The model under review builds one solid part; all positions refer to its coordinate system, in mm. Face numbers are marked on the shaded views. A direction names the side the tool comes from. Give positions to 0.01 mm unless a question says otherwise; leave off trailing zeros. Write each loop counter-clockwise with the first axis right and the second up, starting at its lowest first coordinate (ties: lowest second). Pieces come first, ordered by that corner, then holes. Notation, with made-up numbers: (0.25, 9.25) - (39.25, 9.25) arc R27 ccw to (39.25, 31.25) - close; hole circle Ø7 at (75, 18). An arc over 180 degrees is marked (long way). Write item = value, one per line.
```python
from build123d import *

# Parameters (mm, degrees)
F0_W      = 50.8
F0_H      = 31.75
F1_DEPTH  = 57.15
F2_W      = 50.8
F2_H      = 25.4
F3_DEPTH  = 19.05
F5_DEPTH  = 19.05
F6_DEPTH  = 6.35
F8_DEPTH  = 57.151
F10_DEPTH = 12.701
F12_DEPTH = 12.701
F14_DEPTH = 25.4


with BuildPart() as f1:
    # F0 (on Top) → F1 (new body)
    with BuildSketch(Plane.XY):
        with Locations((25.4, 15.875)):
            Rectangle(F0_W, F0_H)
    extrude(amount=F1_DEPTH)

    # F2 (on face) → F3 (cut)
    with BuildSketch(Plane.XZ):
        with Locations((25.4, 19.05)):
            Rectangle(F2_W, F2_H)
    extrude(amount=-F3_DEPTH, mode=Mode.SUBTRACT)

    # F4 (on face) → F5 (cut)
    with BuildSketch(Plane.XZ):
        with BuildLine():
            ThreePointArc((12.7, 44.45), (16.4197438789, 53.4302561211), (25.4, 57.15))
            Line((25.4, 57.15), (0, 57.15))
            Line((0, 57.15), (0, 44.45))
            Line((0, 44.45), (12.7, 44.45))
        make_face()
        with BuildLine():
            Line((0, 31.75), (25.4, 31.75))
            ThreePointArc((25.4, 31.75), (16.4197438789, 35.4697438789), (12.7, 44.45))
            Line((12.7, 44.45), (0, 44.45))
            Line((0, 44.45), (0, 31.75))
        make_face()
        with BuildLine():
            Line((50.8, 44.45), (38.1, 44.45))
            ThreePointArc((38.1, 44.45), (34.3802561211, 35.4697438789), (25.4, 31.75))
            Line((25.4, 31.75), (50.8, 31.75))
            Line((50.8, 31.75), (50.8, 44.45))
        make_face()
        with BuildLine():
            ThreePointArc((25.4, 57.15), (34.3802561211, 53.4302561211), (38.1, 44.45))
            Line((38.1, 44.45), (50.8, 44.45))
            Line((50.8, 44.45), (50.8, 57.15))
            Line((50.8, 57.15), (25.4, 57.15))
        make_face()
        with BuildLine():
            Line((19.05, 44.45), (31.75, 44.45))
            ThreePointArc((31.75, 44.45), (25.4, 50.8), (19.05, 44.45))
        make_face()
        with BuildLine():
            ThreePointArc((19.05, 44.45), (25.4, 38.1), (31.75, 44.45))
            Line((31.75, 44.45), (19.05, 44.45))
        make_face()
    extrude(amount=-F5_DEPTH, mode=Mode.SUBTRACT)

    # F6 (cut): a face of the model
    f6_faces = [f1.faces().sort_by_distance(p)[0] for p in [
        (25.4, 0, 56.7907897552),
    ]]
    extrude(f6_faces, amount=-F6_DEPTH, mode=Mode.SUBTRACT)

    # F7 (on face) → F8 (cut, through all)
    with BuildSketch(Plane(origin=(0, 0, 0), x_dir=(1, 0, 0), z_dir=(0, 0, -1))):
        with BuildLine():
            Line((0, 0), (0, -12.7))
            ThreePointArc((0, -12.7), (3.7197438789, -3.7197438789), (12.7, 0))
            Line((12.7, 0), (0, 0))
        make_face()
        with BuildLine():
            Line((50.8, 0), (38.1, 0))
            ThreePointArc((38.1, 0), (47.0802561211, -3.7197438789), (50.8, -12.7))
            Line((50.8, -12.7), (50.8, 0))
        make_face()
    extrude(amount=-F8_DEPTH, mode=Mode.SUBTRACT)

    # F9 (on face) → F10 (cut, through all)
    with BuildSketch(Plane.XZ.offset(-19.05)):
        Polygon((12.7, 44.45), (12.7, 57.15), (0, 57.15), (0, 19.05), (12.7, 19.05), align=None)
        Polygon((50.8, 57.15), (38.1, 57.15), (38.1, 44.45), (38.1, 19.05), (50.8, 19.05), align=None)
        with BuildLine():
            Line((38.1, 57.15), (25.4, 57.15))
            ThreePointArc((25.4, 57.15), (34.3802561211, 53.4302561211), (38.1, 44.45))
            Line((38.1, 44.45), (38.1, 57.15))
        make_face()
        with BuildLine():
            Line((25.4, 57.15), (12.7, 57.15))
            Line((12.7, 57.15), (12.7, 44.45))
            ThreePointArc((12.7, 44.45), (16.4197438789, 53.4302561211), (25.4, 57.15))
        make_face()
    extrude(amount=-F10_DEPTH, mode=Mode.SUBTRACT)

    # F11 (on face) → F12 (cut, through all)
    with BuildSketch(Plane.XZ.offset(-19.05)):
        with BuildLine():
            Line((0, 19.05), (0, 6.35))
            ThreePointArc((0, 6.35), (8.9802561211, 10.0697438789), (12.7, 19.05))
            Line((12.7, 19.05), (0, 19.05))
        make_face()
        with BuildLine():
            ThreePointArc((38.1, 19.05), (41.8197438789, 10.0697438789), (50.8, 6.35))
            Line((50.8, 6.35), (50.8, 19.05))
            Line((50.8, 19.05), (38.1, 19.05))
        make_face()
    extrude(amount=-F12_DEPTH, mode=Mode.SUBTRACT)

    # F13 (on face) → F14 (cut)
    with BuildSketch(Plane(origin=(0, 0, 0), x_dir=(1, 0, 0), z_dir=(0, 0, -1))):
        with BuildLine():
            Line((9.525, -9.525), (6.35, -9.525))
            ThreePointArc((6.35, -9.525), (9.525, -12.7), (12.7, -9.525))
            ThreePointArc((12.7, -9.525), (11.7700640303, -7.2799359697), (9.525, -6.35))
            Line((9.525, -6.35), (9.525, -9.525))
        make_face()
        with BuildLine():
            ThreePointArc((9.525, -6.35), (7.2799359697, -7.2799359697), (6.35, -9.525))
            Line((6.35, -9.525), (9.525, -9.525))
            Line((9.525, -9.525), (9.525, -6.35))
        make_face()
        with BuildLine():
            Line((41.275, -9.525), (41.275, -6.35))
            ThreePointArc((41.275, -6.35), (39.0299359697, -11.7700640303), (44.45, -9.525))
            Line((44.45, -9.525), (41.275, -9.525))
        make_face()
        with BuildLine():
            ThreePointArc((44.45, -9.525), (43.5200640303, -7.2799359697), (41.275, -6.35))
            Line((41.275, -6.35), (41.275, -9.525))
            Line((41.275, -9.525), (44.45, -9.525))
        make_face()
    extrude(amount=-F14_DEPTH, mode=Mode.SUBTRACT)


solid = f1.part
```
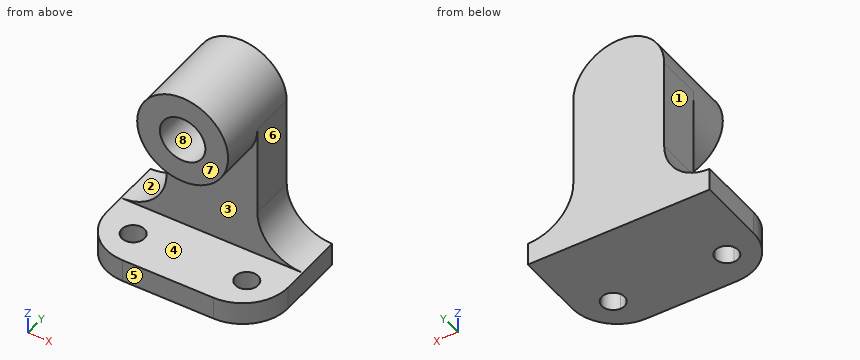
1. For line 1 (Z direction, x = 25.4, y = 10.25); line 2 (X direction, y = 11.5, z = 44.45); line 3 (Z direction, x = 21, y = 7), list the stretches that pass through material, from the lowest coordinate up. Write a range as from..to.
Findings below:
line_1 = 0..6.35, 31.75..38.1, 50.8..57.15
line_2 = 12.7..19.05, 31.75..38.1
line_3 = 0..6.35, 32.54..39.87, 49.03..56.36
2. Take a section at A-A on y = 15. Give the boundary of the cut face in (x, z), and give its area (3 significant figures).
Findings below:
outline = (0, 0) - (50.8, 0) - (50.8, 6.35) - (0, 6.35) - close; circle Ø25.4 at (25.4, 44.45); hole circle Ø12.7 at (25.4, 44.45)
area = 703 mm²
3. Machinability: for the marked faces 4, 5, 6, 7 and 8, which of the approach directions +Z, -Z, +X, -X, +Y, -Y give a long, thin tool a straight path to every point of the face, cutting with its end or side? Answer none if there is none.
Findings below:
face_4 = +X, -X, -Y
face_5 = +Z, -Z, +X, -X, -Y
face_6 = +Z, +X, +Y, -Y
face_7 = +Z, +X, -X, -Y
face_8 = -Y
4. Take a section at C-C on x = 25.4. Give the boundary of the cut face in (y, z), and give its area (3 significant figures).
Findings below:
outline = (0, 0) - (31.75, 0) - (31.75, 57.15) - (6.35, 57.15) - (6.35, 50.8) - (19.05, 50.8) - (19.05, 38.1) - (6.35, 38.1) - (6.35, 31.75) - (19.05, 31.75) - (19.05, 6.35) - (0, 6.35) - close
area = 1,010 mm²
5. Insertion check: P1, Ø4, axis at y = 21.5, z = 28.5, coming from the +X side; P2, Ø10, axis at x = 26.5, z = 45, coming from the -Y side; P3, Ø1, axis at y = 28, z = 49.5, coming from the -X side. Each pin has a flat end and moves straight along its axis. Give the tip position at first contact, or say it passes through.
Findings below:
P1 = 38.1
P2 = 19.05
P3 = 13.54
6. Take a section at D-D on z = 8. Give the boundary of the cut face in (x, y).
Findings below:
outline = (6.26, 19.05) - (44.54, 19.05) - (44.54, 31.75) - (6.26, 31.75) - close
7. Take a section at B-B on x = 43. Give the boundary of the cut face in (y, z).
Findings below:
outline = (0.98, 0) - (6.86, 0) - (6.86, 6.35) - (0.98, 6.35) - close; (12.19, 0) - (31.75, 0) - (31.75, 9.03) - (19.05, 9.03) - (19.05, 6.35) - (12.19, 6.35) - close
8. Draft analysis for pull direction Z (two halves, no side actions). For the marked faces 1, 2 and 3, state which applies: +Z half, -Z half, draft (parallel to the pull), parting line (faces both ways), or undercut.
Findings below:
face_1 = draft
face_2 = +Z half
face_3 = undercut
